Check sheet for the modelled part. Datum: model origin and axes. Units: mm. Round coordinates to 2 decimals unless told otherwise and drop trailing zeros. Order: outer loops, then holes, each group sorted by start corner. A loop starts at its lowest first (then second) coordinate and runs counter-clockwise, first axis right, second up.
(1) Sectioned sample at A-A, the plane z = 127. Enter the section's corners in (x, y) (3 decimals), and give its area (3 significant figures).
(2) Depth check by flat-ended pin: pin 1 (6.5 mm diameter, centred on x = 0, z = -139.7, fed in from -Y); pin 2 (2 mm diameter, centred on x = 6, z = 111.5, fed in from +Y) (3 decimals); pin 3 (6 mm diameter, centred on x = 0, z = 111.125, fed in from -Y); pin 4 (6 mm diameter, centred on x = 0.5, z = -110, fed in from +Y). Enter the tip coordinate at first touch or a pass-through.
(3) Thickness scan on probe 1 along Z at (x, y) = (-6.5, 8.5); probe 2 along X at (y, z) = (11.75, 139.7) (3 decimals); probe 3 along Z at (x, y) = (2, 5.25). Record the ranges inside material, lowest first.
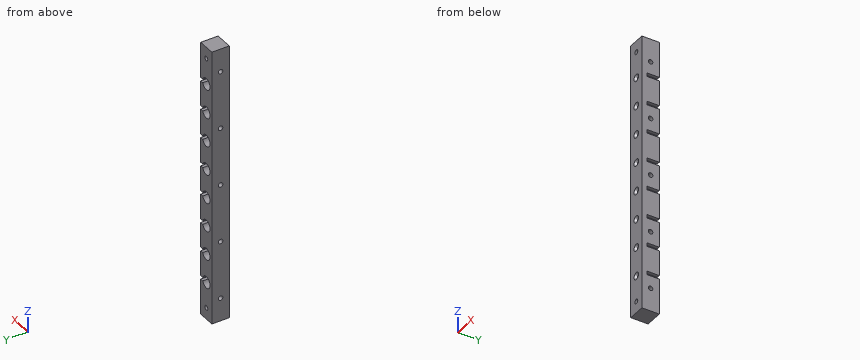
```python
from build123d import *

# Parameters (mm, degrees)
F0_W           = 19.05
F0_H           = 304.8
F1_DEPTH       = 19.05
F3_D           = 5
F5_D           = 3.7973
F5_DEPTH       = 12.7
F5_CSINK_D     = 7.7978
F5_CSINK_ANGLE = 82
F5_TIP         = 1.1408240143
F6_W           = 31.75
F6_H           = 317.5
F6_W_2         = 23.05
F6_H_2         = 308.8
F6_W_3         = 13.335
F6_H_3         = 4
F6_W_4         = 0.9525
F7_DEPTH       = 6.35
F4_R           = 6.35
F8_DEPTH       = 12.7
F10_D          = 5


with BuildPart() as f1:
    # F0 (on Front) → F1 (new body)
    with BuildSketch(Plane.XZ):
        Rectangle(F0_W, F0_H)
    extrude(amount=-F1_DEPTH)

    # F3 (through all)
    with Locations(Plane.YZ.offset(9.525)):
        with Locations((9.525, 127), (9.525, 63.5), (9.525, 0), (9.525, -63.5), (9.525, -127)):
            Hole(F3_D / 2)

    # F5
    with Locations(Plane.XZ):
        with Locations((0, 111.125), (0, 79.375), (0, 47.625), (0, 15.875), (0, -15.875), (0, -47.625), (0, -79.375), (0, -111.125)):
            CounterSinkHole(F5_D / 2, F5_CSINK_D / 2, depth=F5_DEPTH, counter_sink_angle=F5_CSINK_ANGLE)
            with Locations((0, 0, -(F5_DEPTH + F5_TIP / 2))):  # 118° drill point
                Cone(0, F5_D / 2, F5_TIP, mode=Mode.SUBTRACT)

    # F6 (on face) → F7 (cut)
    with BuildSketch(Plane.YZ.offset(9.525)):
        with Locations((9.525, 0)):
            Rectangle(F6_W, F6_H)
        with Locations((9.525, 0)):
            Rectangle(F6_W_2, F6_H_2, mode=Mode.SUBTRACT)
        with Locations((9.525, 0)):
            Rectangle(F6_W_2, F6_H_2)
        Polygon((20.0025, 13.875), (19.05, 13.875), (19.05, -13.875), (20.0025, -13.875), (20.0025, -17.875), (19.05, -17.875), (19.05, -45.625), (20.0025, -45.625), (20.0025, -49.625), (19.05, -49.625), (19.05, -77.375), (20.0025, -77.375), (20.0025, -81.375), (19.05, -81.375), (19.05, -109.125), (20.0025, -109.125), (20.0025, -113.125), (19.05, -113.125), (19.05, -152.4), (0, -152.4), (0, 152.4), (19.05, 152.4), (19.05, 113.125), (20.0025, 113.125), (20.0025, 109.125), (19.05, 109.125), (19.05, 81.375), (20.0025, 81.375), (20.0025, 77.375), (19.05, 77.375), (19.05, 49.625), (20.0025, 49.625), (20.0025, 45.625), (19.05, 45.625), (19.05, 17.875), (20.0025, 17.875), align=None, mode=Mode.SUBTRACT)
        with Locations((12.3825, -15.875)):
            Rectangle(F6_W_3, F6_H_3)
        with Locations((12.3825, 47.625)):
            Rectangle(F6_W_3, F6_H_3)
        with Locations((12.3825, -47.625)):
            Rectangle(F6_W_3, F6_H_3)
        Polygon((5.715, 77.375), (19.05, 77.375), (19.05, 77.3812195068), (19.05, 81.375), (5.715, 81.375), align=None)
        with Locations((12.3825, -79.375)):
            Rectangle(F6_W_3, F6_H_3)
        with Locations((12.3825, -111.125)):
            Rectangle(F6_W_3, F6_H_3)
        with Locations((12.3825, 111.125)):
            Rectangle(F6_W_3, F6_H_3)
        Polygon((5.715, 17.875), (5.715, 13.8770895111), (19.05, 13.8751393007), (19.05, 17.875), align=None)
        with Locations((19.52625, 47.625)):
            Rectangle(F6_W_4, F6_H_3)
        with Locations((19.52625, 111.125)):
            Rectangle(F6_W_4, F6_H_3)
        Polygon((19.05, 17.875), (19.05, 13.8751393007), (20.0025, 13.875), (20.0025, 17.875), align=None)
        Polygon((19.05, 77.3812195068), (20.0025, 77.375), (20.0025, 81.375), (19.05, 81.375), align=None)
    extrude(amount=-F7_DEPTH, mode=Mode.SUBTRACT)

    # F4 (on face) → F8 (cut)
    with BuildSketch(Plane(origin=(0, 19.05, 0), x_dir=(-1, 0, 0), z_dir=(0, 1, 0))):
        with Locations((0, 111.125)):
            Circle(F4_R)
        with Locations((0, 79.375)):
            Circle(F4_R)
        with Locations((0, 47.625)):
            Circle(F4_R)
        with Locations((0, 15.875)):
            Circle(F4_R)
        with Locations((0, -47.625)):
            Circle(F4_R)
        with Locations((0, -79.375)):
            Circle(F4_R)
        with Locations((0, -111.125)):
            Circle(F4_R)
        with Locations((0, -15.875)):
            Circle(F4_R)
    extrude(amount=-F8_DEPTH, mode=Mode.SUBTRACT)

    # F10 (through all)
    with Locations(Plane(origin=(0, 19.05, 0), x_dir=(-1, 0, 0), z_dir=(0, 1, 0))):
        with Locations((0, 139.7), (0, -139.7)):
            Hole(F10_D / 2)


solid = f1.part
```
Derived:
1. outline: (-9.525, 0) - (9.525, 0) - (9.525, 7.025) - (-9.525, 7.025) - close; (-9.525, 12.025) - (9.525, 12.025) - (9.525, 19.05) - (-9.525, 19.05) - close
1. area: 268 mm2
2. pin 1: stops at y = 0
2. pin 2: stops at y = 5.715
2. pin 3: stops at y = 1.03
2. pin 4: stops at y = 6.35
3. probe 1: z = -152.4 to -129.28, -124.72 to -65.78, -61.22 to -2.28, 2.28 to 61.22, 65.78 to 124.72, 129.28 to 152.4
3. probe 2: x = -9.525 to -2.5, 2.5 to 9.525
3. probe 3: z = -152.4 to -141.2, -138.2 to 138.2, 141.2 to 152.4
